from build123d import *

# Parameters (mm, degrees)
F0_R     = 5
F1_ANGLE = -180
F2_DEPTH = 10


with BuildPart() as f1:
    # F0 (on Right) → F1 (revolve)
    with BuildSketch(Plane.YZ):
        with BuildLine():
            Line((-8.539474, 54.358603), (-8.539474, 64.358603))
            Line((-8.539474, 64.358603), (-53.539474, 64.358603))
            Line((-53.539474, 64.358603), (-53.539474, -55.641397))
            Line((-53.539474, -55.641397), (5.460526, -55.641397))
            Line((5.460526, -55.641397), (5.460526, -45.641397))
            Line((5.460526, -45.641397), (5.460526, -45.631396))
            ThreePointArc((5.460526, -45.631396), (-29.246616, -30.641397), (-43.539474, 4.358603))
            ThreePointArc((-43.539474, 4.358603), (-33.850762, 33.939002), (-8.539474, 52.055563))
            Line((-8.539474, 52.055563), (-8.539474, 54.358603))
        make_face()
        with Locations((-43.539474, -45.641397)):
            Circle(F0_R, mode=Mode.SUBTRACT)
        with Locations((-43.539474, 54.358603)):
            Circle(F0_R, mode=Mode.SUBTRACT)
        with Locations((-43.539474, 54.358603)):
            Circle(F0_R)
        with Locations((-43.539474, -45.641397)):
            Circle(F0_R)
    revolve(axis=Axis((0, 6.460526, 9.358603), (0, 0, 1)), revolution_arc=F1_ANGLE)

    # F0 (on Right) → F2 (cut)
    with BuildSketch(Plane.YZ):
        with Locations((-43.539474, 54.358603)):
            Circle(F0_R)
        with Locations((56.460526, 54.358603)):
            Circle(F0_R)
        with Locations((-43.539474, -45.641397)):
            Circle(F0_R)
        with Locations((56.460526, -45.641397)):
            Circle(F0_R)
    extrude(amount=-F2_DEPTH, mode=Mode.SUBTRACT)


solid = f1.part
CAD build for the part. Positions are in the model's coordinates, mm. A direction names the side the tool comes from. Give positions to 0.01 mm unless a question says otherwise; leave off trailing zeros. Return JSON: item names as keys, results as strings.
Item 1: Drop flat-ended pins along their axis: pin 1 (11.5 mm diameter, centred on y = -43.54, z = 54.36, fed in from -X); pin 2 (12 mm diameter, centred on x = -23.5, z = 5.5, fed in from +Y); pin 3 (5 mm diameter, centred on y = 54.5, z = -46.5, fed in from +X); pin 4 (8 mm diameter, centred on y = 54.5, z = 53, fed in from +X). Give the stop position or say it passes through.
Answer below:
{"pin 1": "stops at x = -40.52", "pin 2": "stops at y = 63.85", "pin 3": "stops at x = -10", "pin 4": "stops at x = 0"}
Item 2: Band-saw the part on A-A (x = -6). Give the number of separate pieces and of enclosed holes in the cut face, then the cut area to 3 significant figures.
Answer below:
{"separate pieces": "1", "enclosed holes": "4", "area": "5,970 mm2"}
Item 3: Tool access for faces 1 (the cylindrical face through (-14.996, 6.131, 58.293)), 2 (the flat face through (-30, 6, 64.359)), 3 (the flat face through (-10, -44, 54)): list every direction of +Z, -Z, +X, -X, +Y, -Y with a clear straight run to the whole face (end or side of a thin tool).
Answer below:
{"face 1": "+Z, +X", "face 2": "+Z, +X, -X, +Y, -Y", "face 3": "+X"}
Item 4: Drill centre lines: probe 1 along Z at (x, y) = (-18, -7.5); probe 2 along Y at (x, z) = (-19, -12.5); probe 3 along Z at (x, y) = (-33, -17). Where is each one in solid material? Low to high.
Answer below:
{"probe 1": "z = -55.64 to -40.15, 48.87 to 64.36", "probe 2": "y = -50.45 to -36.61, 49.53 to 63.37", "probe 3": "z = -55.64 to -24.98, 33.69 to 64.36"}
